from build123d import *

# Parameters (mm, degrees)
AUFSATZ_LINEAR_AUSTRAGEN1_DEPTH = 15
AUFSATZ_LINEAR_AUSTRAGEN2_DEPTH = 3
SKIZZE3_8_R                     = 5.5
SCHNITT_LINEAR_AUSTRAGEN1_DEPTH = 3
SKIZZE3_9_R                     = 2.15
SCHNITT_LINEAR_AUSTRAGEN2_DEPTH = 3


with BuildPart() as part:
    # Skizze2 → Aufsatz-Linear austragen1 (new body)
    with BuildSketch(Plane.XY):
        with BuildLine():
            ThreePointArc((-4.1, 0), (0, 4.1), (4.1, 0))
            Line((4.1, 0), (10, 0))
            Line((10, 0), (15, 0))
            Line((15, 0), (15, 3))
            Line((15, 3), (7, 3))
            ThreePointArc((7, 3), (0, 6.657308815), (-7, 3))
            Line((-7, 3), (-15, 3))
            Line((-15, 3), (-15, 0))
            Line((-15, 0), (-10, 0))
            Line((-10, 0), (-4.1, 0))
        make_face()
    extrude(amount=AUFSATZ_LINEAR_AUSTRAGEN1_DEPTH)

    # Skizze3 → Aufsatz-Linear austragen2 (add)
    with BuildSketch(Plane(origin=(0, 3, 0), x_dir=(1, 0, 0), z_dir=(0, 1, 0))):
        with BuildLine():
            ThreePointArc((15, -15), (20.956440423, -7.5), (15, 0))
            Line((15, 0), (15, -15))
        make_face()
        with BuildLine():
            Line((-15, -15), (-15, 0))
            ThreePointArc((-15, 0), (-20.956440423, -7.5), (-15, -15))
        make_face()
    extrude(amount=-AUFSATZ_LINEAR_AUSTRAGEN2_DEPTH)

    # Skizze3<8> → Schnitt-Linear austragen1 (cut)
    with BuildSketch(Plane(origin=(0, 3, 0), x_dir=(1, 0, 0), z_dir=(0, 1, 0))):
        with Locations((-10, -7.5)):
            Circle(SKIZZE3_8_R)
        with Locations((10, -7.5)):
            Circle(SKIZZE3_8_R)
    extrude(amount=SCHNITT_LINEAR_AUSTRAGEN1_DEPTH, mode=Mode.SUBTRACT)

    # Skizze3<9> → Schnitt-Linear austragen2 (cut)
    with BuildSketch(Plane(origin=(0, 3, 0), x_dir=(1, 0, 0), z_dir=(0, 1, 0))):
        with Locations(Location((10, -7.5, 0), (0, 0, 180))):
            Circle(SKIZZE3_9_R)
        with Locations(Location((-10, -7.5, 0), (0, 0, 180))):
            Circle(SKIZZE3_9_R)
    extrude(amount=-SCHNITT_LINEAR_AUSTRAGEN2_DEPTH, mode=Mode.SUBTRACT)


solid = part.part
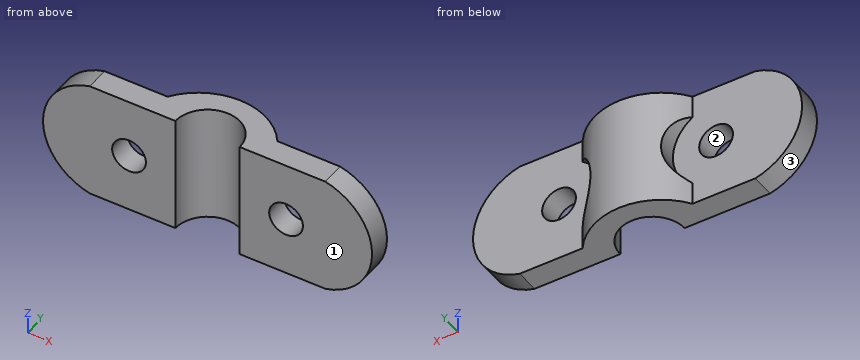
CAD build for the part. Positions are in the model's coordinates, mm. Face numbers are marked on the shaded views. Coordinates: 2 decimals unless noted, no trailing zeros. Loops run counter-clockwise (first coordinate to the right, second up) from the corner with the lowest first, then second, coordinate; pieces in that order, holes last. Notation, with made-up numbers: (42.25, 80) - (90.25, 80) arc R30 cw to (90.25, 111) - close; hole circle Ø4 at (51, 34.25). An arc over 180 degrees is marked (long way). Write item = value, one per line. Start each with the question number.
Q1. Cut at A-A, the plane z = 7.5. List the corners of the cut face in (x, y).
Q2. Cut at C-C, the plane y = 2. List the corners of the cut face in (x, z), then the cut area to 3 significant figures.
Q3. Pull direction Z, two halves, no side cores. Call the marked faces 1, 2 and 3: pulls with the +Z half, pulls with the -Z half, needs draft (parallel to the pull), parting line crosses it, or undercut.
Q4. Drill centre lines: L1, parallel to Z at x = 10, y = 2.1; L2, parallel to Y at x = 16, z = 4.25; L3, parallel to Z at x = 6, y = 3.25. Where is each one in solid material? Low to high.
Q5. Flat gauge pin, fed straight in: pin 1 Ø1.5 at (x, y) = (-13.5, 4.5) entering from -Z. Where does the tip first touch, or does it go through?
Q6. Cut at D-D, the plane z = 4. List the corners of the cut face in (x, y).
Q7. Cut at B-B, the plane x = 10. List the corners of the cut face in (y, z).
Computed:
q1.outline = (-20.96, 0) - (-12.15, 0) - (-12.15, 3) - (-20.96, 3) - close; (-7.85, 0) - (-4.1, 0) arc R4.1 cw to (4.1, 0) - (7.85, 0) - (7.85, 3) - (4.5, 3) - (4.5, 5.37) arc R8.53 ccw to (-4.5, 5.37) - (-4.5, 3) - (-7.85, 3) - close; (12.15, 0) - (20.96, 0) - (20.96, 3) - (12.15, 3) - close
q2.outline = (-15, 0) - (-3.58, 0) - (-3.58, 15) - (-15, 15) arc R7.7 ccw to start; (3.58, 0) - (15, 0) arc R7.7 ccw to (15, 15) - (3.58, 15) - close; hole circle Ø4.3 at (-10, 7.5); hole circle Ø4.3 at (10, 7.5)
q2.area = 447 mm²
q3.face_1 = needs draft
q3.face_2 = undercut
q3.face_3 = parting line crosses it
q4.L1 = 0 to 5.35, 9.65 to 15
q4.L2 = 0 to 3
q4.L3 = 0 to 3.73, 11.27 to 15
q5.pin_1 = through
q6.outline = (-20.12, 0) - (-4.1, 0) arc R4.1 cw to (4.1, 0) - (20.12, 0) - (20.12, 3) - (5.76, 3) - (5.76, 4.42) arc R8.53 ccw to (-5.76, 4.42) - (-5.76, 3) - (-20.12, 3) - close
q7.outline = (0, 0) - (3, 0) - (3, 5.35) - (0, 5.35) - close; (0, 9.65) - (3, 9.65) - (3, 15) - (0, 15) - close
